```python
from build123d import *

# Parameters (mm, degrees)
SKETCH1_R           = 1.5
BOSS_EXTRUDE1_DEPTH = 16
BOSS_EXTRUDE2_DEPTH = 1


with BuildPart() as part:
    # Sketch1 → Boss-Extrude1 (new body)
    with BuildSketch(Plane(origin=(0, 0, 0), x_dir=(0, 0, -1), z_dir=(1, 0, 0))):
        with BuildLine():
            Line((0.49946551, 12.999886025), (-0.50053449, 12.999886025))
            Line((-0.50053449, 12.999886025), (-0.50053449, 1.884665812))
            ThreePointArc((-0.50053449, 1.884665812), (0.000552977, -1.949999922), (0.49946551, 1.88494939))
            Line((0.49946551, 1.88494939), (0.49946551, 12.999886025))
        make_face()
        Circle(SKETCH1_R, mode=Mode.SUBTRACT)
    extrude(amount=BOSS_EXTRUDE1_DEPTH)

    # Sketch2 → Boss-Extrude2 (add)
    with BuildSketch(Plane(origin=(0, 12.999886025, 0), x_dir=(1, 0, 0), z_dir=(0, 1, 0))):
        Polygon((16, -0.50053449), (0, -0.50053449), (0, -30.50053449), (-7.5, -30.50053449), (-7.5, -57.5), (23.5, -57.5), (23.5, -30.50053449), (16, -30.50053449), align=None)
    extrude(amount=-BOSS_EXTRUDE2_DEPTH)


solid = part.part
```
Verification items for the finished model (mm, model axes). A direction names the side the tool comes from. Coordinates: 2 decimals unless noted, no trailing zeros. Loops run counter-clockwise (first coordinate to the right, second up) from the corner with the lowest first, then second, coordinate; pieces in that order, holes last. Notation, with made-up numbers: (-21.5, 35.5) -> (31.5, 35.5) arc R16 cw to (31.5, 41.5) -> close; hole circle Ø8 at (20, -7). An arc over 180 degrees is marked (long way). Answer in a Markdown table with one row per item. Add a question column.
1. Section check C-C, the plane z = 11. Enter the section's corners in (x, y).
2. Draft check along Z on faces 1 (the face through (8, 13, 35)), 2 (the face through (7.89, 0.07, 1.5)), 3 (the face through (8, 7, 0.501)). Enter one of: +Z half, -Z half, draft (parallel to the pull), parting line (faces both ways), or undercut.
3. Section check B-B, the plane x = 4. Enter the section's corners in (y, z).
4. Section check D-D, the plane x = 20.5. Enter the section's corners in (y, z).
5. Material ranges on probe 1 along Y at (x, z) = (7.5, 0); probe 2 along Z at (x, y) = (6.5, 2.75); probe 3 along Y at (x, z) = (20, 33), recorded low to high. Write a range as [from, to].
6. Depth check by flat-ended pin: P1, Ø6, axis at x = 15, y = 1.5, coming from the -Z side; P2, Ø1.5, axis at x = 7, y = 4, coming from the +Z side; P3, Ø5.5, axis at x = 7, y = 6.5, coming from the -Z side; P4, Ø1, axis at x = 18.5, z = 40, coming from the -Y side. Enter the tip coordinate at first touch or a pass-through.
7. Section check A-A, the plane y = 0. Enter the section's corners in (x, z), then the cut area to 3 significant figures.
8. Access from +Z, -Z, +X, -X, +Y, -Y to the whole of each face (thin tool, end or side, straight path). Record for faces 4 (the face through (16, 12.2, 10.7)), 5 (the face through (0, 12.2, 9.4)), 6 (the face through (8, 7, -0.499)), 7 (the face through (7.89, -1.95, 0.08)).
Derived:
| question | item | result |
|---|---|---|
| 1 | outline | (0, 12) -> (16, 12) -> (16, 13) -> (0, 13) -> close |
| 2 | face 1 | draft |
| 2 | face 2 | undercut |
| 2 | face 3 | +Z half |
| 3 | outline | (1.88, -0.5) -> (13, -0.5) -> (13, 57.5) -> (12, 57.5) -> (12, 0.5) -> (1.88, 0.5) arc R1.95 ccw (long way) to start; hole circle Ø3 at (0, 0) |
| 4 | outline | (12, 30.5) -> (13, 30.5) -> (13, 57.5) -> (12, 57.5) -> close |
| 5 | probe 1 | y = [-1.95, -1.5], [1.5, 13] |
| 5 | probe 2 | z = [-0.5, 0.5] |
| 5 | probe 3 | y = [12, 13] |
| 6 | P1 | stops at z = -1.95 |
| 6 | P2 | stops at z = 0.5 |
| 6 | P3 | stops at z = -0.5 |
| 6 | P4 | stops at y = 12 |
| 7 | outline | (0, -1.95) -> (16, -1.95) -> (16, -1.5) -> (0, -1.5) -> close; (0, 1.5) -> (16, 1.5) -> (16, 1.95) -> (0, 1.95) -> close |
| 7 | area | 14.4 mm² |
| 8 | face 4 | -Z, +X, +Y, -Y |
| 8 | face 5 | -Z, -X, +Y, -Y |
| 8 | face 6 | -Z, +X, -X, +Y |
| 8 | face 7 | +X, -X |
